from build123d import *

# Parameters (mm, degrees)
PAD_DEPTH             = 15
POCKET_DEPTH          = 13.5
PAD001_DEPTH          = 15
POLARPATTERN_COUNT    = 3
SKETCH008_R           = 1.6
POCKET001_DEPTH       = 15
POLARPATTERN001_COUNT = 3
SKETCH009_R           = 10
POCKET002_DEPTH       = 5


with BuildPart() as part:
    # Sketch → Pad (new body)
    with BuildSketch(Plane.XY):
        with BuildLine():
            ThreePointArc((0, 24), (-11.489125, -21.071308), (20.174241, 13))
            Line((30.174241, 13), (20.174241, 13))
            Line((30.174241, 24), (30.174241, 13))
            Line((0, 24), (30.174241, 24))
        make_face()
    extrude(amount=PAD_DEPTH)

    # Sketch001 → Pocket (cut)
    with BuildSketch(Plane.XY.offset(15)):
        with BuildLine():
            ThreePointArc((0, 22.5), (-9.486833, -20.402206), (17.204651, 14.5))
            Line((30.174241, 14.5), (17.204651, 14.5))
            Line((30.174241, 22.5), (30.174241, 14.5))
            Line((0, 22.5), (30.174241, 22.5))
        make_face()
    extrude(amount=-POCKET_DEPTH, mode=Mode.SUBTRACT)

    # Sketch007 → Pad001 (new body)
    with BuildSketch(Plane.XY.offset(15)):
        with BuildLine():
            ThreePointArc((25.039208, 7.828671), (26.72977, 12.480769), (22.07767, 14.171327))
            Line((18.658172, 12.574682), (22.07767, 14.171327))
            ThreePointArc((21.61971, 6.232025), (20.38711, 9.519229), (18.658172, 12.574682))
            Line((21.61971, 6.232025), (25.039208, 7.828671))
        make_face()
    pad001 = extrude(amount=-PAD001_DEPTH)

    # PolarPattern: Pad001 ×3 about axis
    polarpattern_axis = Axis((0, 0, 15), (0, 0, 1))
    for i in range(1, POLARPATTERN_COUNT):
        add(pad001.rotate(polarpattern_axis, i * 360 / POLARPATTERN_COUNT))

    # Sketch008 → Pocket001 (cut)
    with BuildSketch(Plane.XY.offset(15)):
        with Locations((23.558442, 11)):
            Circle(SKETCH008_R)
    pocket001 = extrude(amount=-POCKET001_DEPTH, mode=Mode.SUBTRACT)

    # PolarPattern001: Pocket001 ×3 about axis
    polarpattern001_axis = Axis((0, 0, 15), (0, 0, 1))
    for i in range(1, POLARPATTERN001_COUNT):
        add(pocket001.rotate(polarpattern001_axis, i * 360 / POLARPATTERN001_COUNT), mode=Mode.SUBTRACT)

    # Sketch009 → Pocket002 (cut)
    with BuildSketch(Plane(origin=(0, 0, 0), x_dir=(1, 0, 0), z_dir=(0, 0, -1))):
        Circle(SKETCH009_R)
    extrude(amount=-POCKET002_DEPTH, mode=Mode.SUBTRACT)


solid = part.part
Input: part model. Units: mm. Frame: model coordinates. A direction names the side the tool comes from. Give positions to 0.01 mm unless a question says otherwise; leave off trailing zeros. Order: outer loops, then holes, each group sorted by start corner. A loop starts at its lowest first (then second) coordinate and runs counter-clockwise, first axis right, second up. Notation, with made-up numbers: (-6.5, 25) - (2.5, 25) arc R30 cw to (2.5, 57) - close; hole circle Ø7 at (-35.75, 8). An arc over 180 degrees is marked (long way). Answer as a JSON object with one key per item and string values. Group by question number.
Q1. Mould query, pull axis Y, two halves, no side actions, for faces 1 (the face through (24, 14.5, 8)), 2 (the face through (15, 24, 7)), 3 (the face through (9, 8, 0)). Classes: pulls with the +Y half, pulls with the -Y half, needs draft (parallel to the pull), parting line crosses it, or undercut.
Q2. Cut plane B-B, the plane z = 2.75. Output: boundary loops of the cut face in (x, y), then the cut area to 3 significant figures.
Q3. Cut plane D-D, the plane y = -11. Output: boundary loops of the cut face in (x, z).
Q4. Line query: probe 1 along Y at (x, z) = (-3, 9); probe 2 along X at (y, z) = (0, 0.65); probe 3 along Y at (x, z) = (28, 5.25). Output: solid intervals per line, ascending.
Q5. First-contact query: pin 1 Ø8 at (x, z) = (20, 4) entering from -Y; pin 2 Ø13.5 at (x, y) = (5, 1) entering from +Z; pin 3 Ø4 at (x, z) = (16.5, 11.5) entering from -Y. Flat tips, straight axial feed; report the tip coordinate or a pass-through.
Q6. Set-up query: faces 4 (the face through (-22.374, 11.378, 7.605)), 5 (the face through (-2.17, 9.76, 0.74)), 6 (the face through (9, 5, 1.5)), 7 (the face through (15, 22.5, 8)). Return all of +Z, -Z, +X, -X, +Y, -Y with unobstructed straight access to the full face (end or side cutting, diameter ignored); none if empty.
Q7. Cut plane C-C, the plane x = 18. Output: boundary loops of the cut face in (y, z), then the cut area to 3 significant figures.
Q8. Cut plane A-A, the plane y = 0. Output: boundary loops of the cut face in (x, z).
Results:
{
 "1": {"face 1": "undercut", "face 2": "pulls with the +Y half", "face 3": "needs draft"},
 "2": {"outline": "(-23.31, 12.03) - (-21.46, 10.74) arc R24 ccw to (-5.54, -23.35) - (-5.74, -25.6) arc R3.5 ccw to (1.23, -26.21) - (1.43, -23.96) arc R24 ccw to (22.99, 6.87) - (25.04, 7.83) arc R3.5 ccw to (26.43, 13) - (30.17, 13) - (30.17, 14.5) - (17.2, 14.5) arc R22.5 cw to (18.66, 12.57) arc R22.5 cw to (21.62, 6.23) arc R22.5 cw (long way) to (0, 22.5) - (30.17, 22.5) - (30.17, 24) - (0, 24) arc R24 ccw to (-17.45, 16.48) - (-19.3, 17.77) arc R3.5 ccw to start; hole circle Ø3.2 at (-21.31, 14.9); hole circle Ø3.2 at (-2.25, -25.9); hole circle Ø3.2 at (23.56, 11)", "area": "320 mm^2"},
 "3": {"outline": "(-21.33, 0) - (21.33, 0) - (21.33, 15) - (19.63, 15) - (19.63, 1.5) - (-19.63, 1.5) - (-19.63, 15) - (-21.33, 15) - close"},
 "4": {"probe 1": "-29.32 to -27.32, -24.49 to -22.3, 22.3 to 23.81", "probe 2": "-24 to -10, 10 to 24", "probe 3": "13 to 14.5, 22.5 to 24"},
 "5": {"pin 1": "y = -17.89", "pin 2": "z = 1.5", "pin 3": "y = -19.12"},
 "6": {"face 4": "+Z, -Z, -X", "face 5": "+Z, -Z", "face 6": "+Z", "face 7": "+Z, +X"},
 "7": {"outline": "(-15.87, 0) - (24, 0) - (24, 15) - (22.5, 15) - (22.5, 1.5) - (14.5, 1.5) - (14.5, 15) - (13.5, 15) - (13.5, 1.5) - (-13.5, 1.5) - (-13.5, 15) - (-15.87, 15) - close", "area": "126 mm^2"},
 "8": {"outline": "(-24, 0) - (-10, 0) - (-10, 1.5) - (-22.5, 1.5) - (-22.5, 15) - (-24, 15) - close; (10, 0) - (24, 0) - (24, 15) - (22.5, 15) - (22.5, 1.5) - (10, 1.5) - close"}
}
